from build123d import *

# Parameters (mm, degrees)
BOSS_EXTRUDE1_DEPTH = 6.35
SKETCH2_W           = 87.3
SKETCH2_H           = 87.3
CUT_EXTRUDE1_DEPTH  = 6.35
FILLET1_R           = 12.7


with BuildPart() as part:
    # Sketch1 → Boss-Extrude1 (new body)
    with BuildSketch(Plane(origin=(0, 0, 0), x_dir=(1, 0, 0), z_dir=(0, 1, 0))):
        Polygon((-44, 50), (-50, 50), (-50, 44), (-59.5, 44), (-59.5, -44), (-50, -44), (-50, -50), (-44, -50), (-44, -59.5), (44, -59.5), (44, -50), (50, -50), (50, -44), (59.5, -44), (59.5, 44), (50, 44), (50, 50), (44, 50), (44, 59.5), (-44, 59.5), align=None)
    extrude(amount=BOSS_EXTRUDE1_DEPTH)

    # Sketch2 → Cut-Extrude1 (cut)
    with BuildSketch(Plane(origin=(0, 6.35, 0), x_dir=(1, 0, 0), z_dir=(0, 1, 0))):
        Rectangle(SKETCH2_W, SKETCH2_H)
    extrude(amount=-CUT_EXTRUDE1_DEPTH, mode=Mode.SUBTRACT)

    # Fillet1
    fillet1_edges = [part.edges().sort_by_distance(p)[0] for p in [
        (-43.65, 3.175, 43.65),
        (-43.65, 3.175, -43.65),
        (43.65, 3.175, -43.65),
        (43.65, 3.175, 43.65),
    ]]
    fillet(fillet1_edges, radius=FILLET1_R)


solid = part.part
Part model, mm, in its own coordinate system. A direction names the side the tool comes from. Round coordinates to 2 decimals unless told otherwise and drop trailing zeros. Loops run counter-clockwise (first coordinate to the right, second up) from the corner with the lowest first, then second, coordinate; pieces in that order, holes last. Notation, with made-up numbers: (-11, 20.5) - (18, 20.5) arc R9 cw to (18, 31.5) - close; hole circle Ø4 at (27, 38.5). An arc over 180 degrees is marked (long way). Answer as a JSON object with one key per item and string values.
Item 1: Band-saw the part on A-A on y = 2.75. List the corners of the cut face in (x, z), plus the area to 3 significant figures.
Output:
{"outline": "(-59.5, -44) - (-50, -44) - (-50, -50) - (-44, -50) - (-44, -59.5) - (44, -59.5) - (44, -50) - (50, -50) - (50, -44) - (59.5, -44) - (59.5, 44) - (50, 44) - (50, 50) - (44, 50) - (44, 59.5) - (-44, 59.5) - (-44, 50) - (-50, 50) - (-50, 44) - (-59.5, 44) - close; hole (-43.65, -30.95) arc R12.7 ccw to (-30.95, -43.65) - (30.95, -43.65) arc R12.7 ccw to (43.65, -30.95) - (43.65, 30.95) arc R12.7 ccw to (30.95, 43.65) - (-30.95, 43.65) arc R12.7 ccw to (-43.65, 30.95) - close", "area": "5,860 mm2"}
Item 2: Pin check, flat tips, straight feed: pin 1 (1.8 mm diameter, centred on y = 4.5, z = 48, fed in from +X); pin 2 (3 mm diameter, centred on x = -46.5, y = 1.5, fed in from +Z); pin 3 (3 mm diameter, centred on x = 46, y = 2, fed in from -Z). Stop position of each tip, or through.
Output:
{"pin 1": "x = 50", "pin 2": "z = 50", "pin 3": "z = -50"}
Item 3: Tool access for faces 4 (the face through (-44, 3, 55)), 5 (the face through (50, 3, 47)), 6 (the face through (55, 3, -44)), 7 (the face through (39.83, 3.13, 40.03)): list every direction of +Z, -Z, +X, -X, +Y, -Y with a clear straight run to the whole face (end or side of a thin tool).
Output:
{"face 4": "+Z, -X, +Y, -Y", "face 5": "+Z, +X, +Y, -Y", "face 6": "-Z, +X, +Y, -Y", "face 7": "+Y, -Y"}
Item 4: Pull direction X, two halves, no side cores. Call faces 1 (the face through (-50, 3, 47)), 2 (the face through (44, 3, 55)), 3 (the face through (43.65, 3, 0)): pulls with the +X half, pulls with the -X half, needs draft (parallel to the pull), parting line crosses it, or undercut.
Output:
{"face 1": "pulls with the -X half", "face 2": "pulls with the +X half", "face 3": "undercut"}
Item 5: Band-saw the part on D-D on x = 52. List the corners of the cut face in (y, z).
Output:
{"outline": "(0, -44) - (6.35, -44) - (6.35, 44) - (0, 44) - close"}
Item 6: Wall check: L1, parallel to X at y = 5, z = 8.5; L2, parallel to Z at x = -52, y = 4. Give the ranges that are in metal, low to high.
Output:
{"L1": "-59.5 to -43.65, 43.65 to 59.5", "L2": "-44 to 44"}
Item 7: Band-saw the part on C-C on z = -27.5. List the corners of the cut face in (x, y), plus the area to 3 significant figures.
Output:
{"outline": "(-59.5, 0) - (-43.65, 0) - (-43.65, 6.35) - (-59.5, 6.35) - close; (43.65, 0) - (59.5, 0) - (59.5, 6.35) - (43.65, 6.35) - close", "area": "201 mm2"}
Item 8: Band-saw the part on B-B on x = 27. List the corners of the cut face in (y, z), plus the area to 3 significant figures.
Output:
{"outline": "(0, -59.5) - (6.35, -59.5) - (6.35, -43.65) - (0, -43.65) - close; (0, 43.65) - (6.35, 43.65) - (6.35, 59.5) - (0, 59.5) - close", "area": "201 mm2"}
